Verification items for the finished model (mm, model axes). Give positions to 0.01 mm unless a question says otherwise; leave off trailing zeros. Loops run counter-clockwise (first coordinate to the right, second up) from the corner with the lowest first, then second, coordinate; pieces in that order, holes last. Notation, with made-up numbers: (52.5, 39) - (97.5, 39) arc R21 cw to (97.5, 45) - close; hole circle Ø10 at (65.5, 8.25). An arc over 180 degrees is marked (long way). One line per question, with ' | ' between items. Start each with the question number.
1. Thickness scan on line 1 along X through (y, z) = (1.95, -15.75); line 2 along X through (y, z) = (1.6, -68); line 3 along Z through (x, y) = (1, 0.7). Record the ranges inside material, lowest first. Write a range as from..to.
2. Depth check by flat-ended pin: pin 1 Ø6 at (x, z) = (8.5, -44.5) entering from -Y (3 decimals); pin 2 Ø1.2 at (y, z) = (2, -36) entering from +X; pin 3 Ø1.2 at (x, y) = (6, 1.5) entering from +Z. Enter the tip coordinate at first touch or a pass-through.
3. Section check D-D, the plane y = 2.55. Enter the section's corners in (x, z), then the cut area to 3 significant figures.
4. Section check B-B, the plane x = 0. Enter the section's corners in (y, z).
5. Section check A-A, the plane x = 5.5. Enter the section's corners in (y, z), then the cut area to 3 significant figures.
6. Section check C-C, the plane z = -15.75. Enter the section's corners in (x, y), then the cut area to 3 significant figures.
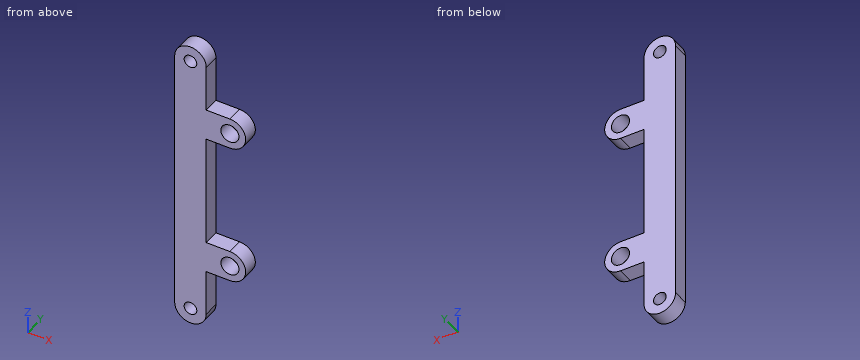
from build123d import *

# Parameters (mm, degrees)
SKETCH1_R           = 1.6
SKETCH1_R_2         = 2.3
BOSS_EXTRUDE1_DEPTH = 4


with BuildPart() as part:
    # Sketch1 → Boss-Extrude1 (new body)
    with BuildSketch(Plane(origin=(0, 0, 0), x_dir=(1, 0, 0), z_dir=(0, 1, 0))):
        with BuildLine():
            Line((-4, 68), (-4, 0))
            ThreePointArc((-4, 0), (0, -4), (4, 0))
            Line((4, 0), (4, 11.75))
            Line((4, 11.75), (10, 11.75))
            ThreePointArc((10, 11.75), (14, 15.75), (10, 19.75))
            Line((10, 19.75), (4, 19.75))
            Line((4, 19.75), (4, 48.25))
            Line((4, 48.25), (10, 48.25))
            ThreePointArc((10, 48.25), (14, 52.25), (10, 56.25))
            Line((10, 56.25), (4, 56.25))
            Line((4, 56.25), (4, 68))
            ThreePointArc((4, 68), (0, 72), (-4, 68))
        make_face()
        with Locations(Location((0, 68, 0), (0, 0, 270))):
            Circle(SKETCH1_R, mode=Mode.SUBTRACT)
        with Locations(Location((0, 0, 0), (0, 0, 270))):
            Circle(SKETCH1_R, mode=Mode.SUBTRACT)
        with Locations(Location((10, 52.25, 0), (0, 0, 270))):
            Circle(SKETCH1_R_2, mode=Mode.SUBTRACT)
        with Locations(Location((10, 15.75, 0), (0, 0, 90))):
            Circle(SKETCH1_R_2, mode=Mode.SUBTRACT)
    extrude(amount=BOSS_EXTRUDE1_DEPTH)


solid = part.part
Results list:
1) line 1: -4..7.7, 12.3..14 | line 2: -4..-1.6, 1.6..4 | line 3: -71.87..-69.25, -66.75..-1.25, 1.25..3.87
2) pin 1: through | pin 2: x = 4 | pin 3: z = -11.75
3) outline: (-4, -68) arc R4 ccw to (4, -68) - (4, -56.25) - (10, -56.25) arc R4 ccw to (10, -48.25) - (4, -48.25) - (4, -19.75) - (10, -19.75) arc R4 ccw to (10, -11.75) - (4, -11.75) - (4, 0) arc R4 ccw to (-4, 0) - close; hole circle Ø3.2 at (0, -68); hole circle Ø3.2 at (0, 0); hole circle Ø4.6 at (10, -52.25); hole circle Ø4.6 at (10, -15.75) | area: 691 mm²
4) outline: (0, -72) - (4, -72) - (4, -69.6) - (0, -69.6) - close; (0, -66.4) - (4, -66.4) - (4, -1.6) - (0, -1.6) - close; (0, 1.6) - (4, 1.6) - (4, 4) - (0, 4) - close
5) outline: (0, -56.25) - (4, -56.25) - (4, -48.25) - (0, -48.25) - close; (0, -19.75) - (4, -19.75) - (4, -11.75) - (0, -11.75) - close | area: 64.0 mm²
6) outline: (-4, 0) - (7.7, 0) - (7.7, 4) - (-4, 4) - close; (12.3, 0) - (14, 0) - (14, 4) - (12.3, 4) - close | area: 53.6 mm²
